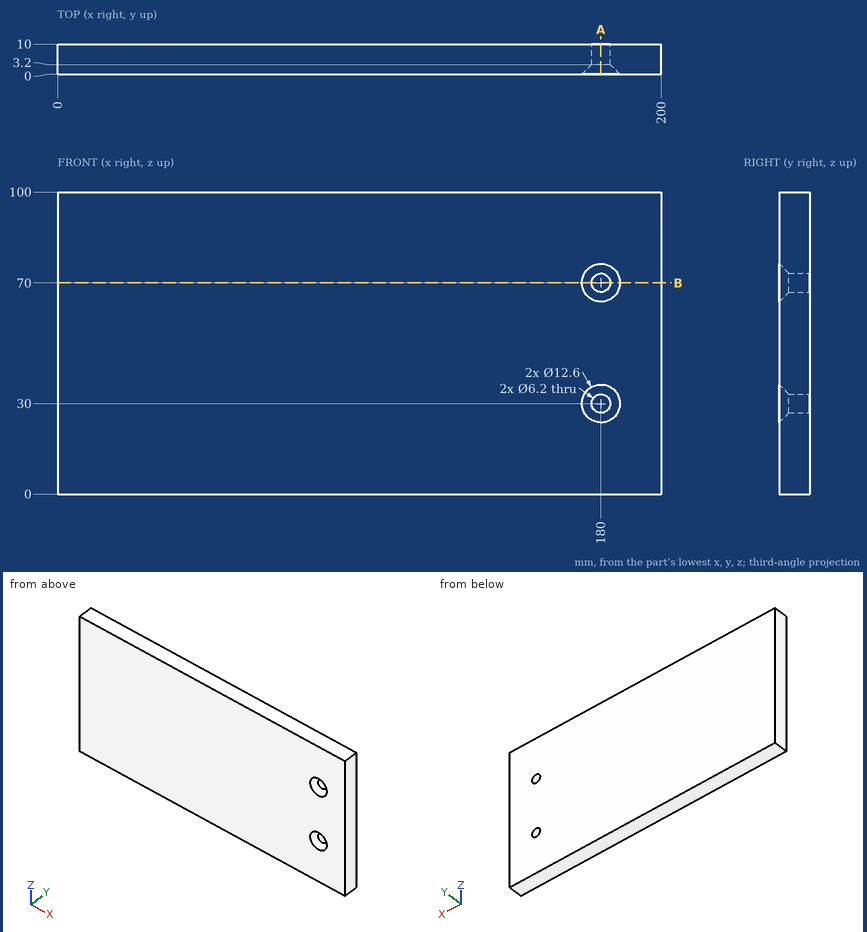
Study the drawing (mm; zero at the part's minimum x, y, z) and answer. Give positions to 0.01 mm unless a question says otherwise; leave off trailing zeros. Order: outer loops, then holes, each group sorted by start corner. A loop starts at its lowest first (then second) coordinate and runs counter-clockwise, first axis right, second up.
1. Straight lines are drawn through the part: L1, parallel to Z at x = 180, y = 7.5; L2, parallel to Z at x = 179, y = 7; L3, parallel to X at y = 8.25, z = 30. For each, find the intervals that lie inside material, in ascending order.
Result sheet:
L1: z = 0 to 26.9, 33.1 to 66.9, 73.1 to 100
L2: z = 0 to 27.07, 32.93 to 67.07, 72.93 to 100
L3: x = 0 to 176.9, 183.1 to 200
2. Section A-A, the plane x = 180 is taken. Determine the outline of the cut face in (y, z).
Result sheet:
outline: (0, 0) - (10, 0) - (10, 26.9) - (3.2, 26.9) - (0, 23.7) - close; (0, 36.3) - (3.2, 33.1) - (10, 33.1) - (10, 66.9) - (3.2, 66.9) - (0, 63.7) - close; (0, 76.3) - (3.2, 73.1) - (10, 73.1) - (10, 100) - (0, 100) - close
3. Section B-B, the plane z = 70 is taken. Determine the outline of the cut face in (x, y), and give its area (3 significant figures).
Result sheet:
outline: (0, 0) - (173.7, 0) - (176.9, 3.2) - (176.9, 10) - (0, 10) - close; (183.1, 3.2) - (186.3, 0) - (200, 0) - (200, 10) - (183.1, 10) - close
area: 1,930 mm2
